```python
from build123d import *

# Parameters (mm, degrees)
SKETCH1_R           = 5
BOSS_EXTRUDE1_DEPTH = 5
SKETCH2_R           = 2
CUT_EXTRUDE1_DEPTH  = 86


with BuildPart() as part:
    # Sketch1 → Boss-Extrude1 (new body)
    with BuildSketch(Plane.XY):
        Polygon((0, 0), (40, 0), (40, 20), (60, 20), (60, 60), (0, 60), align=None)
        with Locations((18, 42)):
            Circle(SKETCH1_R, mode=Mode.SUBTRACT)
    extrude(amount=BOSS_EXTRUDE1_DEPTH)

    # Sketch2 → Cut-Extrude1 (cut, through all)
    with BuildSketch(Plane(origin=(0, 0, 0), x_dir=(-1, 0, 0), z_dir=(0, 0, -1))):
        with Locations((-50, 32)):
            Circle(SKETCH2_R)
        with Locations((-28, 10)):
            Circle(SKETCH2_R)
    extrude(amount=-CUT_EXTRUDE1_DEPTH, mode=Mode.SUBTRACT)


solid = part.part
```
Part model, mm, in its own coordinate system. A direction names the side the tool comes from. Give positions to 0.01 mm unless a question says otherwise; leave off trailing zeros. Order: outer loops, then holes, each group sorted by start corner. A loop starts at its lowest first (then second) coordinate and runs counter-clockwise, first axis right, second up. Notation, with made-up numbers: M 62.25,58.25 L 96.25,58.25 A33 cw 96.25,94.25 Z; hole C 62,0 d9. An arc over 180 degrees is marked long. Use a Markdown table: item, result. Add a question column.
(1) Saw through at A-A, the plane y = 32. Give the cut face in (x, z), and give its area (3 significant figures).
(2) 3-axis set-ups, long thin cutter, end or side, ignore diameter. For faces 4 (the face through (30, 30, 0)), 5 (the face through (50, 20, 2)): which of +Z, -Z, +X, -X, +Y, -Y reach the whole face in a straight line?
(3) Drop flat-ended pins along their axis: P1, Ø6, axis at x = 51.5, y = 26, coming from the -Z side; P2, Ø3, axis at y = 17, z = 1, coming from the +X side. Give the stop position or say it passes through.
(4) Saw through at B-B, the plane z = 2.15. Give the cut face in (x, y), and give its area (3 significant figures).
(5) Probe line 1 along Y through (x, z) = (28, 0.2); line 2 along Y through (x, z) = (50, 1.1); line 3 along X through (y, z) = (31.5, 3.05). List the from-to ranges inside material, lowest first. Write a range as [from, to].
(6) Saw through at D-D, the plane x = 53. Give the cut face in (y, z).
(7) Mould opens along X. For faces 1 (the face through (0, 30, 2)), 2 (the face through (50, 30, 2)), 3 (the face through (20, 0, 2)) say: +X half, -X half, draft (parallel to the pull), parting line (faces both ways), or undercut.
(8) Saw through at C-C, the plane x = 18. Give the cut face in (y, z), and give its area (3 significant figures).
Answer key:
| question | item | result |
|---|---|---|
| 1 | outline | M 0,0 L 48,0 L 48,5 L 0,5 Z; M 52,0 L 60,0 L 60,5 L 52,5 Z |
| 1 | area | 280 mm^2 |
| 2 | face 4 | -Z, +X, -X, +Y, -Y |
| 2 | face 5 | +Z, -Z, +X, -Y |
| 3 | P1 | z = 0 |
| 3 | P2 | x = 40 |
| 4 | outline | M 0,0 L 40,0 L 40,20 L 60,20 L 60,60 L 0,60 Z; hole C 18,42 d10; hole C 28,10 d4; hole C 50,32 d4 |
| 4 | area | 3,100 mm^2 |
| 5 | line 1 | [0, 8], [12, 60] |
| 5 | line 2 | [20, 30], [34, 60] |
| 5 | line 3 | [0, 48.06], [51.94, 60] |
| 6 | outline | M 20,0 L 60,0 L 60,5 L 20,5 Z |
| 7 | face 1 | -X half |
| 7 | face 2 | undercut |
| 7 | face 3 | draft |
| 8 | outline | M 0,0 L 37,0 L 37,5 L 0,5 Z; M 47,0 L 60,0 L 60,5 L 47,5 Z |
| 8 | area | 250 mm^2 |
